Work out the finished part from the listing and answer in its coordinate system (mm). Face numbers are marked on the shaded views. A direction names the side the tool comes from. Round coordinates to 2 decimals unless told otherwise and drop trailing zeros. Order: outer loops, then holes, each group sorted by start corner. A loop starts at its lowest first (then second) coordinate and runs counter-clockwise, first axis right, second up. Notation, with made-up numbers: (-12, 78) -> (27, 78) arc R13 cw to (27, 102) -> close; hole circle Ø4 at (67.5, 61). An arc over 180 degrees is marked (long way). Use a Markdown table: item, result. Add a question column.
Item 1: A tool of negligible diameter and unlimited length cuts with its end or side. For the marked faces 1 and 2, from which of +Z, -Z, +X, -X, +Y, -Y can it reach the whole face along a straight path? Write none if from no direction.
Item 2: A cutting plane is placed at B-B, the plane y = -71. Determine the outline of the cut face in (x, z).
Item 3: A cutting plane is placed at A-A, the plane y = -37. Determine the outline of the cut face in (x, z), plus the area to 3 significant figures.
Item 4: Find the intervals of material crossed by L1, parallel to Y at x = 27, z = 104; L2, parallel to Z at x = 51, y = -39; L3, parallel to X at y = 33, z = 91.5, in increasing order. Write a range as [from, to].
Item 5: Flat-ended cylindrical pins translate along their axes: P1, Ø12, axis at x = -20.5, z = 74, coming from the -Y side; P2, Ø12, axis at y = -156, z = 32, coming from the -X side; P3, Ø3, axis at x = -43.5, y = -57.5, coming from the -Z side (3 decimals). Find the tip coordinate at first contact, or state that the pin passes through.
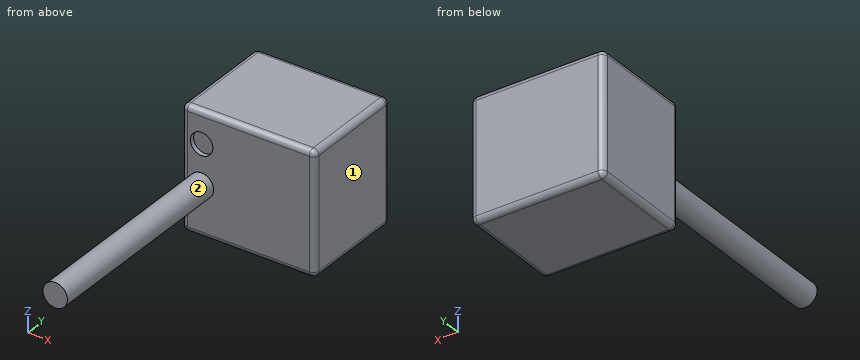
from build123d import *

# Parameters (mm, degrees)
F0_W     = 120.674577
F0_H     = 96.105173
F1_DEPTH = 110.744
F2_T     = -2.54
F3_W     = 115.594577
F3_H     = 105.664
F4_DEPTH = 4.064
F6_D     = 20.32
F6_DEPTH = 5.08
F7_R     = 11.07788
F8_DEPTH = 188.214
F9_R     = 5.08


with BuildPart() as f1:
    # F0 (on Top) → F1 (new body)
    with BuildSketch(Plane.XY):
        with Locations((-2.504403, 2.655324)):
            Rectangle(F0_W, F0_H)
    extrude(amount=F1_DEPTH)

    # F2
    f2_openings = [f1.faces().sort_by_distance(p)[0] for p in [
        (-2.504403, -45.397263, 55.372),
    ]]
    offset(amount=F2_T, openings=f2_openings)

    # F3 (on face) → F4 (join)
    with BuildSketch(Plane.XZ.offset(45.397263)):
        with Locations((-2.504403, 55.372)):
            Rectangle(F3_W, F3_H)
    extrude(amount=-F4_DEPTH)

    # F6
    with Locations(Plane.XZ.offset(45.397263)):
        with Locations((-44.790465, 81.706673)):
            Hole(F6_D / 2, depth=F6_DEPTH)

    # F7 (on face) → F8 (join)
    with BuildSketch(Plane.XZ.offset(45.397263)):
        with Locations((-44.997666, 45.472905)):
            Circle(F7_R)
    extrude(amount=F8_DEPTH)

    # F9
    f9_edges = [f1.edges().sort_by_distance(p)[0] for p in [
        (-2.504403, -45.397263, 110.744),
        (57.832886, -45.397263, 55.372),
        (57.832886, 50.70791, 55.372),
        (57.832886, 2.655324, 110.744),
        (-2.504403, 50.70791, 110.744),
        (-62.841691, 2.655324, 110.744),
        (-62.841691, -45.397263, 55.372),
        (-2.504403, -45.397263, 0),
        (57.832886, 2.655324, 0),
        (-2.504403, 50.70791, 0),
        (-62.841691, 2.655324, 0),
        (-62.841691, 50.70791, 55.372),
    ]]
    fillet(f9_edges, radius=F9_R)


solid = f1.part
Reported:
| question | item | result |
|---|---|---|
| 1 | face 1 | +Z, -Z, +X, +Y, -Y |
| 1 | face 2 | -Y |
| 2 | outline | circle Ø22.16 at (-45, 45.47) |
| 3 | outline | (-62.84, 5.08) arc R5.08 ccw to (-57.76, 0) -> (52.75, 0) arc R5.08 ccw to (57.83, 5.08) -> (57.83, 105.66) arc R5.08 ccw to (52.75, 110.74) -> (-57.76, 110.74) arc R5.08 ccw to (-62.84, 105.66) -> close; hole (-60.3, 2.54) -> (55.29, 2.54) -> (55.29, 108.2) -> (-60.3, 108.2) -> close |
| 3 | area | 1,130 mm² |
| 4 | L1 | [-45.4, -41.33], [48.17, 50.71] |
| 4 | L2 | [0, 2.54], [108.2, 110.74] |
| 4 | L3 | [-62.84, -60.3], [55.29, 57.83] |
| 5 | P1 | y = -45.4 |
| 5 | P2 | x = -53.18 |
| 5 | P3 | z = 34.395 |
